Autodesk Inventor part; units mm, degrees
ref_plane "作業平面1" through (0, 0, 0) normal (0, 1, 0) x (-1, 0, 0)
ref_plane "YZ Plane" through (0, 0, 0) normal (1, 0, 0) x (0, 1, 0)
ref_plane "XZ Plane" through (0, 0, 0) normal (0, 1, 0) x (-1, 0, 0)
sketch "スケッチ1" plane through (0, 0, 0) normal (0, 0, 1) x (1, 0, 0)
  circle A0 centre (0, 0) radius 1.5
  circle A1 centre (0, 0) radius 2.5
  line L0 (0, 0) -> (0, 2.5)
  dimension "d1" = 5
  dimension "d0" = 3
extrude "押し出し1" add sketch "スケッチ1" along normal blind 14 contours A0 | A1
extrude "押し出し2" add sketch "スケッチ1" against normal blind 18.5 contours A0
ref_plane "作業平面1" through (0, 0, 0) normal (0, 1, 0) x (-1, 0, 0)
sketch "スケッチ2" plane through (0, 0, 0) normal (0, 1, 0) x (-1, 0, 0)
  line L0 (2.5, 14) -> (-2.5, 14)
  circle A0 centre (0, 14) radius 4.75
  point P0 (0, 0)
  dimension "d6" = 9.5
extrude "押し出し3" add sketch "スケッチ2" along normal mid plane 4
sketch "スケッチ3" plane through (0, 2, 0) normal (0, 1, 0) x (1, 0, 0)
  line L0 (-1.5, -14) -> (1.5, -14)
  circle A0 centre (0, -14) radius 4.75
  point P0 (0, 0)
  dimension "d9" = 9.5
extrude "押し出し4" cut sketch "スケッチ3" along normal blind 4
sketch "スケッチ4" plane through (0, -2, 0) normal (0, -1, 0) x (1, 0, 0)
  line L0 (1.5, 14) -> (-1.5, 14)
  circle A0 centre (0, 14) radius 4.75
  point P0 (0, 0)
  dimension "d12" = 9.5
extrude "押し出し5" cut sketch "スケッチ4" along normal blind 4
hole "穴1" at (0, -2, 14) direction (0, 1, 0) diameter 3 end through all
sketch "スケッチ5" plane through (0, 0, 0) normal (0, 0, -1) x (-1, 0, 0)
  circle A0 centre (0, 0) radius 2.5
  circle A1 centre (0, 0) radius 1.5
properties part number "ダンパー下パーツ"
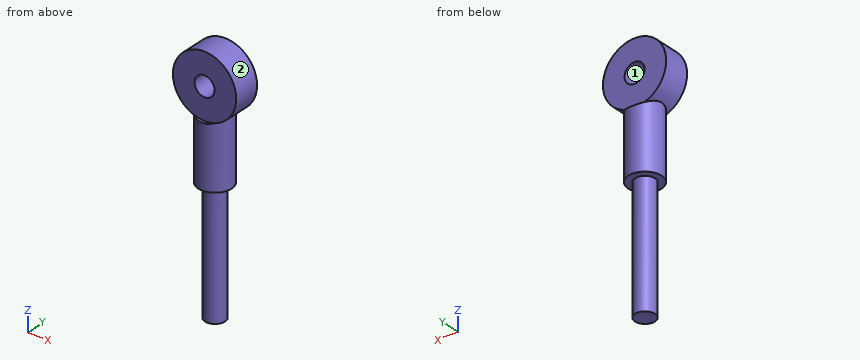
Could you check a few things on this model? Use its own coordinates, in mm. Face numbers are marked on the shaded views. Round coordinates to 2 decimals unless told otherwise and drop trailing zeros. Write each loop counter-clockwise with the first axis right and the second up, starting at its lowest first coordinate (ties: lowest second). Pieces come first, ordered by that corner, then holes. Notation, with made-up numbers: (1.25, -35) -> (29.25, -35) arc R24 ccw to (29.25, -10) -> close; hole circle Ø7 at (67.25, -35.75). An arc over 180 degrees is marked (long way). Use a Markdown table: item, result.
1. If we section it at C-C (z = 14): List the corners of the cut face in (x, y) for me, then the cut area to 3 significant figures.
Answer key:
| item | result |
|---|---|
| outline | (-4.75, -2) -> (-1.5, -2) -> (-1.5, 2) -> (-4.75, 2) -> close; (1.5, -2) -> (4.75, -2) -> (4.75, 2) -> (1.5, 2) -> close |
| area | 26.0 mm^2 |
2. Please list where these lines run through material, in increasing order: probe 1 along X at (y, z) = (-1.15, 14); probe 2 along Z at (x, y) = (0, 1.05); probe 3 along Y at (x, z) = (-2, 1.5).
Answer key:
| item | result |
|---|---|
| probe 1 | x = -4.75 to -1.5, 1.5 to 4.75 |
| probe 2 | z = -18.5 to 12.5, 15.5 to 18.75 |
| probe 3 | y = -1.5 to 1.5 |
3. If we section it at D-D (z = -3): List the corners of the cut face in (x, y) for me, then the cut area to 3 significant figures.
Answer key:
| item | result |
|---|---|
| outline | circle Ø3 at (0, 0) |
| area | 7.07 mm^2 |
4. If we section it at A-A (y = 0): List the corners of the cut face in (x, z) for me.
Answer key:
| item | result |
|---|---|
| outline | (-2.5, 0) -> (-1.5, 0) -> (-1.5, -18.5) -> (1.5, -18.5) -> (1.5, 0) -> (2.5, 0) -> (2.5, 9.96) arc R4.75 ccw (long way) to (-2.5, 9.96) -> close; hole circle Ø3 at (0, 14) |
5. For pin 1 Ø3 at (x, z) = (-3, 4.5) entering from -Y; pin 2 Ø4 at (x, z) = (-3, 10) entering from +Y; pin 3 Ø1 at (y, z) = (-1, 13.5) entering from +X; pin 4 Ø5 at (x, z) = (-2, -14.5) entering from -Y, each with a flat end and sliding along its axis, tell me the tip position at first contact or that it passes through.
Answer key:
| item | result |
|---|---|
| pin 1 | stops at y = -2 |
| pin 2 | stops at y = 2.25 |
| pin 3 | stops at x = 4.75 |
| pin 4 | stops at y = -1.5 |
6. We'd pull the mould along X, two halves only. Please class the marked faces 1 and 2: +X half, -X half, draft (parallel to the pull), parting line (faces both ways), or undercut.
Answer key:
| item | result |
|---|---|
| face 1 | undercut |
| face 2 | parting line |
7. If we section it at B-B (x = 0): List the corners of the cut face in (y, z) for me, then the cut area to 3 significant figures.
Answer key:
| item | result |
|---|---|
| outline | (-2.5, 0) -> (-1.5, 0) -> (-1.5, -18.5) -> (1.5, -18.5) -> (1.5, 0) -> (2.5, 0) -> (2.5, 9.25) -> (2, 9.25) -> (2, 12.5) -> (-2, 12.5) -> (-2, 9.25) -> (-2.5, 9.25) -> close; (-2, 15.5) -> (2, 15.5) -> (2, 18.75) -> (-2, 18.75) -> close |
| area | 128 mm^2 |
